Geometry check sheet. Reference: the model listing, model coordinates, mm. Round coordinates to 2 decimals unless told otherwise and drop trailing zeros. Write each loop counter-clockwise with the first axis right and the second up, starting at its lowest first coordinate (ties: lowest second). Pieces come first, ordered by that corner, then holes. Notation, with made-up numbers: M -16.75,-13 L 8.25,-13 A16 cw 8.25,13 Z; hole C -9,-32.75 d8. An arc over 180 degrees is marked long. Answer as CSV lines item,"result". Start each with the question number.
```python
from build123d import *

# Parameters (mm, degrees)
SKETCH1_W           = 300
SKETCH1_H           = 120
SKETCH1_W_2         = 40
SKETCH1_H_2         = 12.7
BOSS_EXTRUDE1_DEPTH = 12.7
SKETCH2_W           = 42.7
SKETCH2_H           = 35
CUT_EXTRUDE1_DEPTH  = 12.7
SKETCH3_W           = 40
SKETCH3_H           = 12.7
CUT_EXTRUDE2_DEPTH  = 12.7
SKETCH4_W           = 40
SKETCH4_H           = 12.7
CUT_EXTRUDE3_DEPTH  = 12.7


with BuildPart() as part:
    # Sketch1 → Boss-Extrude1 (new body)
    with BuildSketch(Plane(origin=(0, 0, 0), x_dir=(0, 0, -1), z_dir=(1, 0, 0))):
        Rectangle(SKETCH1_W, SKETCH1_H)
        with Locations((0, -66.35)):
            Rectangle(SKETCH1_W_2, SKETCH1_H_2)
    extrude(amount=BOSS_EXTRUDE1_DEPTH)

    # Sketch2 → Cut-Extrude1 (cut)
    with BuildSketch(Plane(origin=(12.7, 0, 0), x_dir=(0, 0, -1), z_dir=(1, 0, 0))):
        with Locations((-128.65, -42.5)):
            Rectangle(SKETCH2_W, SKETCH2_H)
        with Locations((128.65, -42.5)):
            Rectangle(SKETCH2_W, SKETCH2_H)
    extrude(amount=-CUT_EXTRUDE1_DEPTH, mode=Mode.SUBTRACT)

    # Sketch3 → Cut-Extrude2 (cut)
    with BuildSketch(Plane(origin=(12.7, 0, 0), x_dir=(0, 0, -1), z_dir=(1, 0, 0))):
        with Locations((0, 53.65)):
            Rectangle(SKETCH3_W, SKETCH3_H)
    extrude(amount=-CUT_EXTRUDE2_DEPTH, mode=Mode.SUBTRACT)

    # Sketch4 → Cut-Extrude3 (cut)
    with BuildSketch(Plane(origin=(12.7, 0, 0), x_dir=(0, 0, -1), z_dir=(1, 0, 0))):
        with Locations((-80, 53.65)):
            Rectangle(SKETCH4_W, SKETCH4_H)
    extrude(amount=-CUT_EXTRUDE3_DEPTH, mode=Mode.SUBTRACT)


solid = part.part
```
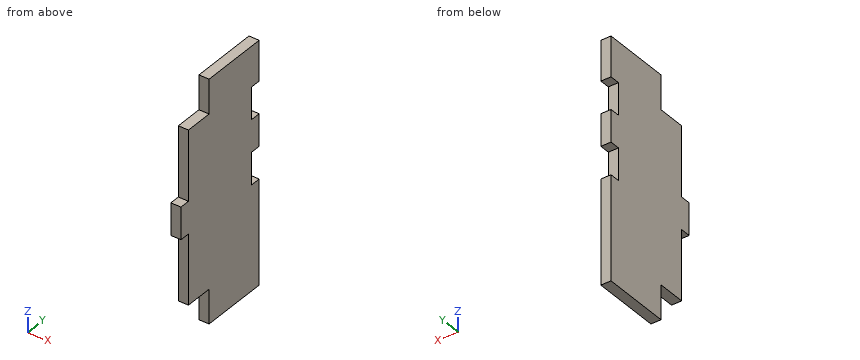
1) Section check C-C, the plane y = -37.5. Record the cut outline in (x, z).
2) Scan lines: line 1 (Z direction, x = 8.25, y = 50); line 2 (Z direction, x = 1.75, y = -67); line 3 (Z direction, x = 8.75, y = -51). Record each from-to range of solid material in increasing order. Write a range as from..to.
3) Section check A-A, the plane x = 5. Record the cut outline in (y, z).
4) Go/stop test with flat-tipped pins: pin 1 (6.5 mm diameter, centred on x = 5.5, y = -48.5, fed in from -Z); pin 2 (3 mm diameter, centred on x = 10, z = -34.5, fed in from -Y); pin 3 (6.5 mm diameter, centred on x = 7, z = -138, fed in from -Y). Record where each tip stops, or that it passes through.
5) Section check B-B, the plane z = 66.5. Record the cut outline in (x, y).
Results:
1,outline,"M 0,-107.3 L 12.7,-107.3 L 12.7,107.3 L 0,107.3 Z"
2,line 1,"z = -150..-20, 20..60, 100..150"
2,line 2,"z = -20..20"
2,line 3,"z = -107.3..107.3"
3,outline,"M -72.7,-20 L -60,-20 L -60,-107.3 L -25,-107.3 L -25,-150 L 60,-150 L 60,-20 L 47.3,-20 L 47.3,20 L 60,20 L 60,60 L 47.3,60 L 47.3,100 L 60,100 L 60,150 L -25,150 L -25,107.3 L -60,107.3 L -60,20 L -72.7,20 Z"
4,pin 1,"stops at z = -107.3"
4,pin 2,"stops at y = -60"
4,pin 3,"stops at y = -25"
5,outline,"M 0,-60 L 12.7,-60 L 12.7,47.3 L 0,47.3 Z"
